The listing builds one solid part. Answer for the finished solid, in the listing's coordinates (mm). A direction names the side the tool comes from. Round coordinates to 2 decimals unless told otherwise and drop trailing zeros. Write each loop counter-clockwise with the first axis right and the second up, starting at its lowest first coordinate (ties: lowest second). Pieces come first, ordered by that corner, then holes. Notation, with made-up numbers: (28.25, 41) - (62.25, 41) arc R16 ccw to (62.25, 59) - close; hole circle Ø5 at (-38, 4). An arc over 180 degrees is marked (long way). Use a Markdown table: item, result. Add a question column.
1) A cutting plane is placed at B-B (y = 10). Give the vertices of the cut face in (x, z).
2) Each of these flat-tipped pins is pushed along its axis until it touches: P1, Ø3, axis at x = -178, y = 15, coming from the +Z side; P2, Ø4, axis at y = 21, z = 25, coming from the -X side; P3, Ø5, axis at y = -7.5, z = 15, coming from the +X side; P4, Ø6, axis at x = -179.5, z = -26, coming from the +Y side. Where does it stop, or does it pass through?
3) A tool of negligible diameter and unlimited length cuts with its end or side. For faces 5 (the cylindrical face through (-176.427, 15.821, 20.633)), 6 (the cylindrical face through (-180.575, -12.165, 13.267)), from which of +Z, -Z, +X, -X, +Y, -Y can it reach the whole face along a straight path? Write none if from no direction.
4) A cutting plane is placed at A-A (z = 0). Give the vertices of the cut face in (x, y), then the cut area to 3 significant figures.
5) A cutting plane is placed at D-D (z = -32.5). Give the vertices of the cut face in (x, y), then the cut area to 3 significant figures.
6) Determine the mould class of faces 1 (the cylindrical face through (-181.14, -1.4, 34.69)), 2 (the cylindrical face through (-181.14, 34.69, 1.4)), 3 (the flat face through (-181.906, 17, -17)), 4 (the cylindrical face through (-184.19, -6.31, -20.03)) for opening direction Y: +Y half, -Y half, draft (parallel to the pull), parting line (faces both ways), or undercut.
7) Find the intervals of material crossed by probe 1 along Y at (x, z) = (-181.5, 0); probe 2 along X at (y, z) = (14.5, 19.5); probe 3 along Z at (x, y) = (-179.5, -1), in increasing order. Write a range as from..to.
```python
from build123d import *

# Parameters (mm, degrees)
CSK_FOR_M5_COUNTERSUNK_FLAT_HEAD_SCREW1_D           = 5.2
CSK_FOR_M5_COUNTERSUNK_FLAT_HEAD_SCREW1_CSINK_D     = 10.1
CSK_FOR_M5_COUNTERSUNK_FLAT_HEAD_SCREW1_CSINK_ANGLE = 90
CIRPATTERN1_COUNT                                   = 4


with BuildPart() as part:
    # Sketch2 → Revolve1 (revolve)
    with BuildSketch(Plane.XY, mode=Mode.PRIVATE) as revolve1_sk:
        Polygon((-174.905599099, 26), (-177.905599099, 26), (-177.905599099, 40), (-181.905599099, 40), (-181.905599099, 21), (-186.405599099, 21), (-186.405599099, 18), (-174.905599099, 18), align=None)
    revolve(revolve1_sk.sketch.rotate(Axis((0, 0, 0), (-1, 0, 0)), 90), axis=Axis((0, 0, 0), (-1, 0, 0)))

    # CSK for M5 Countersunk Flat Head Screw1 (through all)
    with Locations(Plane(origin=(-177.905599099, 0, 0), x_dir=(0, 0, -1), z_dir=(1, 0, 0))):
        with Locations((0, 32.5)):
            csk_for_m5_countersunk_flat_head_screw1 = CounterSinkHole(CSK_FOR_M5_COUNTERSUNK_FLAT_HEAD_SCREW1_D / 2, CSK_FOR_M5_COUNTERSUNK_FLAT_HEAD_SCREW1_CSINK_D / 2, counter_sink_angle=CSK_FOR_M5_COUNTERSUNK_FLAT_HEAD_SCREW1_CSINK_ANGLE)

    # CirPattern1: CSK for M5 Countersunk Flat Head Screw1 ×4 about axis
    cirpattern1_axis = Axis((0, 0, 0), (1, 0, 0))
    for i in range(1, CIRPATTERN1_COUNT):
        add(csk_for_m5_countersunk_flat_head_screw1.rotate(cirpattern1_axis, i * 360 / CIRPATTERN1_COUNT), mode=Mode.SUBTRACT)


solid = part.part
```
Entries:
| question | item | result |
|---|---|---|
| 1 | outline | (-186.41, -18.47) - (-181.91, -18.47) - (-181.91, -38.73) - (-177.91, -38.73) - (-177.91, -24) - (-174.91, -24) - (-174.91, -14.97) - (-186.41, -14.97) - close; (-186.41, 14.97) - (-174.91, 14.97) - (-174.91, 24) - (-177.91, 24) - (-177.91, 38.73) - (-181.91, 38.73) - (-181.91, 18.47) - (-186.41, 18.47) - close |
| 2 | P1 | stops at z = 37.65 |
| 2 | P2 | stops at x = -181.91 |
| 2 | P3 | stops at x = -174.91 |
| 2 | P4 | stops at y = 32.73 |
| 3 | face 5 | +X |
| 3 | face 6 | +X, -X |
| 4 | outline | (-186.41, -21) - (-181.91, -21) - (-181.91, -29.9) - (-180.36, -29.9) - (-177.91, -27.45) - (-177.91, -26) - (-174.91, -26) - (-174.91, -18) - (-186.41, -18) - close; (-186.41, 18) - (-174.91, 18) - (-174.91, 26) - (-177.91, 26) - (-177.91, 27.45) - (-180.36, 29.9) - (-181.91, 29.9) - (-181.91, 21) - (-186.41, 21) - close; (-181.91, -40) - (-177.91, -40) - (-177.91, -37.55) - (-180.36, -35.1) - (-181.91, -35.1) - close; (-181.91, 35.1) - (-180.36, 35.1) - (-177.91, 37.55) - (-177.91, 40) - (-181.91, 40) - close |
| 4 | area | 197 mm² |
| 5 | outline | (-181.91, -23.32) - (-177.91, -23.32) - (-177.91, -5.05) - (-180.36, -2.6) - (-181.91, -2.6) - close; (-181.91, 2.6) - (-180.36, 2.6) - (-177.91, 5.05) - (-177.91, 23.32) - (-181.91, 23.32) - close |
| 5 | area | 160 mm² |
| 6 | face 1 | undercut |
| 6 | face 2 | undercut |
| 6 | face 3 | draft |
| 6 | face 4 | parting line |
| 7 | probe 1 | y = -40..-35.1, -29.9..-18, 18..29.9, 35.1..40 |
| 7 | probe 2 | x = -181.91..-174.91 |
| 7 | probe 3 | z = -39.99..-35.81, -29.19..-17.97, 17.97..29.19, 35.81..39.99 |
